Input: part model. Units: mm. Frame: model coordinates. Face numbers are marked on the shaded views. A direction names the side the tool comes from. Give positions to 0.01 mm unless a question says otherwise; leave off trailing zeros. Order: outer loops, then holes, each group sorted by start corner. A loop starts at its lowest first (then second) coordinate and runs counter-clockwise, first axis right, second up. Notation, with made-up numbers: M 26,50.25 L 47,50.25 A23 ccw 47,74.25 Z; hole C 68,-37 d10. An arc over 180 degrees is marked long. Use a Markdown table: item, result.
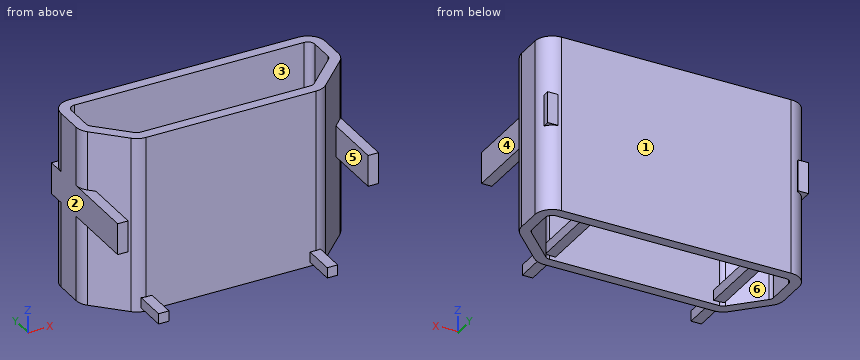
from build123d import *

# Parameters (mm, degrees)
EXTRUDE_1_DEPTH     = 5.06
CUT_EXTRUDE_1_REACH = 7.06
SKETCH_2_W          = 0.3
SKETCH_2_H          = 0.3
SKETCH_2_H_2        = 0.9
EXTRUDE_2_DEPTH     = 3.5


with BuildPart() as part:
    # 草图1 → 凸台-拉伸1 (new body)
    with BuildSketch(Plane.XY):
        with BuildLine():
            Line((-3.603553391, 0.953553391), (-2.796446609, 0.146446609))
            ThreePointArc((-2.796446609, 0.146446609), (-2.634234935, 0.038060234), (-2.442893219, 0))
            Line((-2.442893219, 0), (2.442893219, 0))
            ThreePointArc((2.442893219, 0), (2.634234935, 0.038060234), (2.796446609, 0.146446609))
            Line((2.796446609, 0.146446609), (3.703553391, 1.053553391))
            ThreePointArc((3.703553391, 1.053553391), (3.811939766, 1.215765065), (3.85, 1.407106781))
            Line((3.85, 1.407106781), (3.85, 2.1))
            ThreePointArc((3.85, 2.1), (3.703553391, 2.453553391), (3.35, 2.6))
            Line((3.35, 2.6), (-3.25, 2.6))
            ThreePointArc((-3.25, 2.6), (-3.603553391, 2.453553391), (-3.75, 2.1))
            Line((-3.75, 2.1), (-3.75, 1.307106781))
            ThreePointArc((-3.75, 1.307106781), (-3.711939766, 1.115765065), (-3.603553391, 0.953553391))
        make_face()
    extrude(amount=EXTRUDE_1_DEPTH)

    # 草图4 → 切除-拉伸1 (cut, up to next)
    with BuildSketch(Plane(origin=(0, 0, 0), x_dir=(-1, 0, 0), z_dir=(0, 0, -1)), mode=Mode.PRIVATE) as cut_extrude_1_sk1:
        with BuildLine():
            Line((-2.442893219, 0.3), (2.442893219, 0.3))
            ThreePointArc((2.442893219, 0.3), (2.519429905, 0.315224093), (2.584314575, 0.358578644))
            Line((2.584314575, 0.358578644), (3.391421356, 1.165685425))
            ThreePointArc((3.391421356, 1.165685425), (3.434775907, 1.230570095), (3.45, 1.307106781))
            Line((3.45, 1.307106781), (3.45, 2.1))
            ThreePointArc((3.45, 2.1), (3.391421356, 2.241421356), (3.25, 2.3))
            Line((3.25, 2.3), (-3.35, 2.3))
            ThreePointArc((-3.35, 2.3), (-3.491421356, 2.241421356), (-3.55, 2.1))
            Line((-3.55, 2.1), (-3.55, 1.407106781))
            ThreePointArc((-3.55, 1.407106781), (-3.534775907, 1.330570095), (-3.491421356, 1.265685425))
            Line((-3.491421356, 1.265685425), (-2.584314575, 0.358578644))
            ThreePointArc((-2.584314575, 0.358578644), (-2.519429905, 0.315224093), (-2.442893219, 0.3))
        make_face()
    cut_extrude_1_tool1 = extrude(cut_extrude_1_sk1.sketch, amount=-CUT_EXTRUDE_1_REACH, mode=Mode.PRIVATE) & part.part
    add(cut_extrude_1_tool1.solids().sort_by_distance((0.027478, 1.348077, 0))[0], mode=Mode.SUBTRACT)

    # 草图2 → 凸台-拉伸2 (add)
    with BuildSketch(Plane(origin=(0, 2.6, 0), x_dir=(1, 0, 0), z_dir=(0, 1, 0))):
        with Locations((-2.425, -0.26)):
            Rectangle(SKETCH_2_W, SKETCH_2_H)
        with Locations((-3.6, -2.91)):
            Rectangle(SKETCH_2_W, SKETCH_2_H_2)
        with Locations((3.6, -2.91)):
            Rectangle(SKETCH_2_W, SKETCH_2_H_2)
        with Locations((2.425, -0.26)):
            Rectangle(SKETCH_2_W, SKETCH_2_H)
    extrude(amount=-EXTRUDE_2_DEPTH)


solid = part.part
1) Cut plane C-C on x = 0.5. Return loops of the section in (y, z).
Response values:
| item | result |
|---|---|
| outline | M 0,0 L 0.3,0 L 0.3,5.06 L 0,5.06 Z; M 2.3,0 L 2.6,0 L 2.6,5.06 L 2.3,5.06 Z |
2) Cut plane D-D on y = 0.55. Return loops of the section in (x, z) (3 decimals), and give its area (3 significant figures).
Response values:
| item | result |
|---|---|
| outline | M -3.75,2.46 L -3.45,2.46 L -3.45,3.36 L -3.75,3.36 Z; M -3.2,0 L -2.776,0 L -2.776,5.06 L -3.2,5.06 Z; M -2.575,0.11 L -2.275,0.11 L -2.275,0.41 L -2.575,0.41 Z; M 2.275,0.11 L 2.575,0.11 L 2.575,0.41 L 2.275,0.41 Z; M 2.776,0 L 3.2,0 L 3.2,5.06 L 2.776,5.06 Z; M 3.45,2.46 L 3.75,2.46 L 3.75,3.36 L 3.45,3.36 Z |
| area | 5.01 mm² |
3) Cut plane B-B on z = 0.6. Return loops of the section in (x, y), and give its area (3 significant figures).
Response values:
| item | result |
|---|---|
| outline | M -3.75,1.31 A0.5 ccw -3.6,0.95 L -2.8,0.15 A0.5 ccw -2.44,0 L 2.44,0 A0.5 ccw 2.8,0.15 L 3.7,1.05 A0.5 ccw 3.85,1.41 L 3.85,2.1 A0.5 ccw 3.35,2.6 L -3.25,2.6 A0.5 ccw -3.75,2.1 Z; hole M -3.45,1.31 A0.2 ccw -3.39,1.17 L -2.58,0.36 A0.2 ccw -2.44,0.3 L 2.44,0.3 A0.2 ccw 2.58,0.36 L 3.49,1.27 A0.2 ccw 3.55,1.41 L 3.55,2.1 A0.2 ccw 3.35,2.3 L -3.25,2.3 A0.2 ccw -3.45,2.1 Z |
| area | 5.28 mm² |
4) Material intervals for line 1 (X direction, y = 2, z = 0.3) (3 decimals); line 2 (X direction, y = -0.3, z = 2.8); line 3 (Y direction, x = 0, z = 4.8), sorted ascending. Write a range as from..to.
Response values:
| item | result |
|---|---|
| line 1 | x = -3.75..-3.45, -2.575..-2.275, 2.275..2.575, 3.55..3.85 |
| line 2 | x = -3.75..-3.45, 3.45..3.75 |
| line 3 | y = 0..0.3, 2.3..2.6 |
5) First-contact query: pin 1 Ø2 at (x, z) = (1.5, 4) entering from -Y; pin 2 Ø1.5 at (x, y) = (3, 0.5) entering from -Z. Flat tips, straight axial feed; report the tip coordinate or a pass-through.
Response values:
| item | result |
|---|---|
| pin 1 | stops at y = 0 |
| pin 2 | stops at z = 0 |
6) Reachability of the marked faces 4, 5 and 6 from +Z, -Z, +X, -X, +Y, -Y: full face, straight path, thin tool, end or side. Return the list, or none.
Response values:
| item | result |
|---|---|
| face 4 | +Z, -Z, +X, -Y |
| face 5 | +Z, -Z, -Y |
| face 6 | +Z, -Z |
7) Cut plane A-A on y = -0.2. Return loops of the section in (x, z) (3 decimals).
Response values:
| item | result |
|---|---|
| outline | M -3.75,2.46 L -3.45,2.46 L -3.45,3.36 L -3.75,3.36 Z; M -2.575,0.11 L -2.275,0.11 L -2.275,0.41 L -2.575,0.41 Z; M 2.275,0.11 L 2.575,0.11 L 2.575,0.41 L 2.275,0.41 Z; M 3.45,2.46 L 3.75,2.46 L 3.75,3.36 L 3.45,3.36 Z |
8) Mould query, pull axis Y, two halves, no side actions, for the marked faces 1, 2 and 3. Classes: released by +Y, released by -Y, zero draft, split by the parting line, or undercut.
Response values:
| item | result |
|---|---|
| face 1 | released by +Y |
| face 2 | zero draft |
| face 3 | undercut |
